```python
from build123d import *

# Parameters (mm, degrees)
F1_DEPTH = 40
F2_W     = 10
F2_H     = 30
F3_DEPTH = 20
F4_R     = 5
F5_DEPTH = 30.001
F6_W     = 30
F6_H     = 10
F7_DEPTH = 20
F8_R     = 5
F9_DEPTH = 10.001


with BuildPart() as f1:
    # F0 (on Front) → F1 (new body)
    with BuildSketch(Plane.XZ):
        Polygon((-5.380323, 14.753425), (-5.380323, 4.753425), (24.619677, 4.753425), (24.619677, 34.753425), (14.619677, 34.753425), (14.619677, 14.753425), align=None)
    extrude(amount=-F1_DEPTH)

    # F2 (on face) → F3 (join)
    with BuildSketch(Plane.YZ.offset(24.619677)):
        with Locations((35, 19.753425)):
            Rectangle(F2_W, F2_H)
    extrude(amount=F3_DEPTH)

    # F4 (on face) → F5 (cut, through all)
    with BuildSketch(Plane.YZ.offset(24.619677)):
        with Locations((15, 24.753425)):
            Circle(F4_R)
    extrude(amount=-F5_DEPTH, mode=Mode.SUBTRACT)

    # F6 (on face) → F7 (join)
    with BuildSketch(Plane(origin=(-5.380323, 0, 0), x_dir=(0, -1, 0), z_dir=(-1, 0, 0))):
        with Locations((-25, 9.753425)):
            Rectangle(F6_W, F6_H)
    extrude(amount=F7_DEPTH)

    # F8 (on face) → F9 (cut, through all)
    with BuildSketch(Plane.XY.offset(14.753425)):
        with Locations((-10.380323, 25)):
            Circle(F8_R)
    extrude(amount=-F9_DEPTH, mode=Mode.SUBTRACT)


solid = f1.part
```
Work out the finished part from the listing and answer in its coordinate system (mm). A direction names the side the tool comes from. Coordinates: 2 decimals unless noted, no trailing zeros. Loops run counter-clockwise (first coordinate to the right, second up) from the corner with the lowest first, then second, coordinate; pieces in that order, holes last.
1) Flat-ended cylindrical pins translate along their axes: pin 1 (10 mm diameter, centred on x = 30, y = 23, fed in from -Z); pin 2 (13 mm diameter, centred on y = 15, z = 24.75, fed in from -X); pin 3 (6 mm diameter, centred on x = 31, z = 23.5, fed in from -Y); pin 4 (5 mm diameter, centred on x = -16.5, z = 9, fed in from -Y). Find the tip coordinate at first contact, or state that the pin passes through.
Results:
pin 1: passes through
pin 2: stops at x = 14.62
pin 3: stops at y = 30
pin 4: stops at y = 10
2) Section A-A (y = 25) is taken. Give the vertices of the cut face in (x, z).
Results:
outline: (-25.38, 4.75) - (-15.38, 4.75) - (-15.38, 14.75) - (-25.38, 14.75) - close; (-5.38, 4.75) - (24.62, 4.75) - (24.62, 34.75) - (14.62, 34.75) - (14.62, 14.75) - (-5.38, 14.75) - close
3) Consider probe 1 along X at (y, z) = (8, 26.5); probe 2 along X at (y, z) = (3.5, 6.75); probe 3 along Y at (x, z) = (27, 14.5). Determine where each line is inside the solid, lowest interval first.
Results:
probe 1: x = 14.62 to 24.62
probe 2: x = -5.38 to 24.62
probe 3: y = 30 to 40
4) Section B-B (x = -8.5) is taken. Give the vertices of the cut face in (y, z).
Results:
outline: (10, 4.75) - (20.37, 4.75) - (20.37, 14.75) - (10, 14.75) - close; (29.63, 4.75) - (40, 4.75) - (40, 14.75) - (29.63, 14.75) - close
5) For a pull along Y with two mould halves and no side action, classify faces 5 (the cylindrical face through (-11.46, 20.12, 9.82)), 6 (the flat face through (24.62, 14.8, 19.5)), 7 (the flat face through (16, 0, 17)) as +Y half, -Y half, draft (parallel to the pull), parting line (faces both ways), or undercut.
Results:
face 5: undercut
face 6: draft
face 7: -Y half
6) For faces 1 (the flat face through (-15, 10, 10)), 2 (the flat face through (34, 30, 20)), 3 (the flat face through (-5, 20, 14.753)), 4 (the flat face through (23, 24, 34.753)), determine the directions among +Z, -Z, +X, -X, +Y, -Y from which every point of the face is accessible in a straight line to the end or side of a thin tool.
Results:
face 1: +Z, -Z, -X, -Y
face 2: +Z, -Z, +X, -Y
face 3: +Z, -X, +Y, -Y
face 4: +Z, +X, -X, +Y, -Y
7) Section D-D (z = 10.25) is taken. Give the vertices of the cut face in (x, y), plus the area to 3 significant figures.
Results:
outline: (-25.38, 10) - (-5.38, 10) - (-5.38, 0) - (24.62, 0) - (24.62, 30) - (44.62, 30) - (44.62, 40) - (-25.38, 40) - close; hole circle Ø10 at (-10.38, 25)
area: 1,920 mm2
8) Section C-C (z = 23.75) is taken. Give the vertices of the cut face in (x, y).
Results:
outline: (14.62, 0) - (24.62, 0) - (24.62, 10.1) - (14.62, 10.1) - close; (14.62, 19.9) - (24.62, 19.9) - (24.62, 30) - (44.62, 30) - (44.62, 40) - (14.62, 40) - close
